from build123d import *

# Parameters (mm, degrees)
SKETCH1_W                                       = 10
SKETCH1_H                                       = 20
BOSS_EXTRUDE1_DEPTH                             = 5
BOSS_EXTRUDE2_DEPTH                             = 28
M5_CLEARANCE_HOLE1_D                            = 5.5
M5_CLEARANCE_HOLE1_DEPTH                        = 10
M5_CLEARANCE_HOLE1_TIP                          = 1.652366702
CSK_FOR_M4_FLAT_HEAD_MACHINE_SCREW1_D           = 5.1
CSK_FOR_M4_FLAT_HEAD_MACHINE_SCREW1_DEPTH       = 15
CSK_FOR_M4_FLAT_HEAD_MACHINE_SCREW1_CSINK_D     = 5.5
CSK_FOR_M4_FLAT_HEAD_MACHINE_SCREW1_CSINK_ANGLE = 70
CSK_FOR_M4_FLAT_HEAD_MACHINE_SCREW1_TIP         = 1.532194579
FILLET1_R                                       = 0.5
M3_START                                        = -5
M3_CLEARANCE_SLOT1_DEPTH                        = 5


# Read off the part's stored shape, not the designer's step: M3 Clearance Slot1
with BuildPart() as part:
    # Sketch1 → Boss-Extrude1 (new body)
    with BuildSketch(Plane(origin=(0, 0, 0), x_dir=(1, 0, 0), z_dir=(0, 1, 0))):
        Polygon((0, 20), (0, 0), (12.002075382, 0), (12.002075382, 5), (27.002075382, 5), (20, 15), (50, 15), (42.997924618, 5), (57.997924618, 5), (57.997924618, 0), (70, 0), (70, 20), align=None)
        with Locations((-5, 10)):
            Rectangle(SKETCH1_W, SKETCH1_H)
        Polygon((12.002075382, 5), (12.002075382, 0), (57.997924618, 0), (57.997924618, 5), (42.997924618, 5), (50, 15), (20, 15), (27.002075382, 5), align=None)
        with Locations((75, 10)):
            Rectangle(SKETCH1_W, SKETCH1_H)
    extrude(amount=BOSS_EXTRUDE1_DEPTH)

    # Sketch1<3> → Boss-Extrude2 (add)
    with BuildSketch(Plane(origin=(0, 0, 0), x_dir=(1, 0, 0), z_dir=(0, 1, 0))):
        Polygon((12.002075382, 5), (12.002075382, 0), (57.997924618, 0), (57.997924618, 5), (42.997924618, 5), (50, 15), (20, 15), (27.002075382, 5), align=None)
    extrude(amount=BOSS_EXTRUDE2_DEPTH)

    # M5 Clearance Hole1
    with Locations(Plane(origin=(0, 5, 0), x_dir=(1, 0, 0), z_dir=(0, 1, 0))):
        with Locations((75, 10), (-5, 10)):
            Hole(M5_CLEARANCE_HOLE1_D / 2, depth=M5_CLEARANCE_HOLE1_DEPTH)
            with Locations((0, 0, -(M5_CLEARANCE_HOLE1_DEPTH + M5_CLEARANCE_HOLE1_TIP / 2))):  # 118° drill point
                Cone(0, M5_CLEARANCE_HOLE1_D / 2, M5_CLEARANCE_HOLE1_TIP, mode=Mode.SUBTRACT)

    # CSK for M4 Flat Head Machine Screw1
    with Locations(Plane(origin=(0, 28, 0), x_dir=(1, 0, 0), z_dir=(0, 1, 0))):
        with Locations((35, 9.9)):
            CounterSinkHole(CSK_FOR_M4_FLAT_HEAD_MACHINE_SCREW1_D / 2, CSK_FOR_M4_FLAT_HEAD_MACHINE_SCREW1_CSINK_D / 2, depth=CSK_FOR_M4_FLAT_HEAD_MACHINE_SCREW1_DEPTH, counter_sink_angle=CSK_FOR_M4_FLAT_HEAD_MACHINE_SCREW1_CSINK_ANGLE)
            with Locations((0, 0, -(CSK_FOR_M4_FLAT_HEAD_MACHINE_SCREW1_DEPTH + CSK_FOR_M4_FLAT_HEAD_MACHINE_SCREW1_TIP / 2))):  # 118° drill point
                Cone(0, CSK_FOR_M4_FLAT_HEAD_MACHINE_SCREW1_D / 2, CSK_FOR_M4_FLAT_HEAD_MACHINE_SCREW1_TIP, mode=Mode.SUBTRACT)

    # Fillet1
    fillet1_edges = [part.edges().sort_by_distance(p)[0] for p in [
        (12.002075382, 16.5, -5),
        (57.997924618, 16.5, -5),
        (50, 16.5, -15),
        (20, 16.5, -15),
    ]]
    fillet(fillet1_edges, radius=FILLET1_R)

    # M3 Clearance Slot1 outline → M3 Clearance Slot1 (cut)
    with BuildSketch(Plane.XY.offset(M3_START)):
        with BuildLine():
            Line((54.697924618, 8.835678671), (54.697924618, 20.435678671))
            ThreePointArc((54.697924618, 20.435678671), (52.997924618, 22.135678671), (51.297924618, 20.435678671))
            Line((51.297924618, 20.435678671), (51.297924618, 8.835678671))
            ThreePointArc((51.297924618, 8.835678671), (52.997924618, 7.135678671), (54.697924618, 8.835678671))
        make_face()
        with BuildLine():
            Line((18.702075382, 8.835678671), (18.702075382, 20.435678671))
            ThreePointArc((18.702075382, 20.435678671), (17.002075382, 22.135678671), (15.302075382, 20.435678671))
            Line((15.302075382, 20.435678671), (15.302075382, 8.835678671))
            ThreePointArc((15.302075382, 8.835678671), (17.002075382, 7.135678671), (18.702075382, 8.835678671))
        make_face()
    extrude(amount=M3_CLEARANCE_SLOT1_DEPTH, mode=Mode.SUBTRACT)


solid = part.part
Could you check a few things on this model? Use its own coordinates, in mm. A direction names the side the tool comes from. Give positions to 0.01 mm unless a question says otherwise; leave off trailing zeros. Order: outer loops, then holes, each group sorted by start corner. A loop starts at its lowest first (then second) coordinate and runs counter-clockwise, first axis right, second up. Notation, with made-up numbers: (61.25, 65.25) - (110.25, 65.25) arc R16 cw to (110.25, 82.25) - close; hole circle Ø7 at (-2.75, 44.5). An arc over 180 degrees is marked (long way). Return JSON: item names as keys, results as strings. Group by question number.
Q1. Suppose I cut it at B-B, the plane z = -3. Please give me the cut outline in (x, y), and give its area (3 significant figures).
Q2. Will these pins go through, and if not, where does the flat tip stop? pin 1 Ø2.5 at (y, z) = (12.5, -2.5) entering from -X; pin 2 Ø1.5 at (y, z) = (13, -2.5) entering from +X; pin 3 Ø6 at (y, z) = (9.5, -10.5) entering from +X.
Q3. Suppose I cut it at A-A, the plane x = -5. Please give me the cut outline in (y, z).
Q4. Thinking about a two-plate mould opening in Z: for faces 1 (the face through (54.698, 15, -3)), 2 (the face through (35.409, 11.734, -9.73)), 3 (the face through (35, 16, -15)), which applies, pulls with the +Z half, pulls with the -Z half, needs draft (parallel to the pull), parting line crosses it, or undercut?
Q5. Please list where these lines run through material, in increasing order: line 1 along X through (y, z) = (2.4, -10); line 2 along X through (y, z) = (13, -3.25); line 3 along Z through (x, y) = (-5, 1.45). Write a range as [from, to].
Q6. Suppose I cut it at C-C, the plane y = 6. Please give me the cut outline in (x, z).
Q7. Which directions (+Z, -Z, +X, -X, +Y, -Y) give clear straight access to the entire face, cutting with the end or side of a thin tool? Please do faces 4 (the face through (37.548, 20.254, -10.012)), 5 (the face through (57.998, 16, -2)), 6 (the face through (20, 16, -5)), 7 (the face through (15.302, 15, -3)).
Q8. Suppose I cut it at D-D, the plane x = 53.5. Please give me the cut outline in (y, z), and give its area (3 significant figures).
Resolved:
{
 "1": {"outline": "(-10, 0) - (80, 0) - (80, 5) - (58, 5) - (58, 28) - (12, 28) - (12, 5) - (-10, 5) - close; hole (15.3, 8.84) arc R1.7 ccw to (18.7, 8.84) - (18.7, 20.44) arc R1.7 ccw to (15.3, 20.44) - close; hole (51.3, 8.84) arc R1.7 ccw to (54.7, 8.84) - (54.7, 20.44) arc R1.7 ccw to (51.3, 20.44) - close", "area": "1,410 mm2"},
 "2": {"pin 1": "stops at x = 12", "pin 2": "stops at x = 58", "pin 3": "stops at x = 48.95"},
 "3": {"outline": "(0, -20) - (5, -20) - (5, -12.75) - (0, -12.75) - close; (0, -7.25) - (5, -7.25) - (5, 0) - (0, 0) - close"},
 "4": {"face 1": "needs draft", "face 2": "undercut", "face 3": "pulls with the -Z half"},
 "5": {"line 1": "x = [-10, -7.75], [-2.25, 72.25], [77.75, 80]", "line 2": "x = [12, 15.3], [18.7, 51.3], [54.7, 58]", "line 3": "z = [-20, -12.75], [-7.25, 0]"},
 "6": {"outline": "(12, -4.5) arc R0.5 ccw to (12.5, -5) - (27, -5) - (20.55, -14.21) arc R0.5 ccw to (20.96, -15) - (49.04, -15) arc R0.5 ccw to (49.45, -14.21) - (43, -5) - (57.5, -5) arc R0.5 ccw to (58, -4.5) - (58, 0) - (12, 0) - close"},
 "7": {"face 4": "+Y", "face 5": "+Z, -Z, +X, +Y", "face 6": "-X, +Y", "face 7": "+Z, -Z"},
 "8": {"outline": "(0, -20) - (5, -20) - (5, -5) - (7.21, -5) - (7.21, 0) - (0, 0) - close; (22.06, -5) - (28, -5) - (28, 0) - (22.06, 0) - close", "area": "141 mm2"}
}
